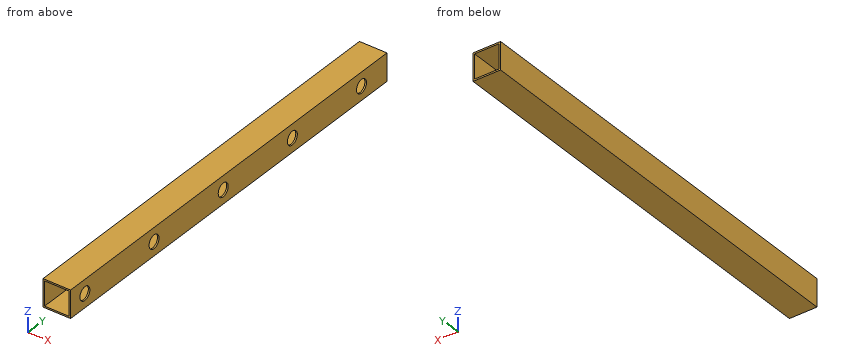
Autodesk Inventor part; units mm, degrees
ref_plane "YZ Plane" through (0, 0, 0) normal (1, 0, 0) x (0, 1, 0)
ref_plane "XZ Plane" through (0, 0, 0) normal (0, 1, 0) x (-1, 0, 0)
ref_plane "XY Plane" through (0, 0, 0) normal (0, 0, 1) x (1, 0, 0)
sketch "Sketch9" plane through (0, 0, 0) normal (0, 1, 0) x (-1, 0, 0)
  line L0 (17.5, 17.5) -> (-17.5, 17.5)
  line L1 (-17.5, 17.5) -> (-17.5, -17.5)
  line L2 (-17.5, -17.5) -> (17.5, -17.5)
  line L3 (17.5, -17.5) -> (17.5, 17.5)
  line L4 (17.5, 17.5) -> (-17.5, -17.5) construction
  line L5 (-17.5, 17.5) -> (17.5, -17.5) construction
  line L6 (-15.5, 15.5) -> (15.5, 15.5)
  line L7 (15.5, 15.5) -> (15.5, -15.5)
  line L8 (15.5, -15.5) -> (-15.5, -15.5)
  line L9 (-15.5, -15.5) -> (-15.5, 15.5)
  point P0 (0, 0)
  dimension "d172" = 35
  dimension "d173" = 35
  dimension "d174" = 2
extrude "Extrusion3" add sketch "Sketch9" against normal blind 540
sketch "Sketch10" plane through (0, 0, 0) normal (1, 0, 0) x (0, 1, 0)
  line L0 (0, 17.5) -> (0, -17.5) construction
  line L1 (0, 17.5) -> (-540, 17.5) construction
  line L2 (-540, -17.5) -> (-540, 17.5) construction
  line L3 (0, -17.5) -> (-540, -17.5) construction
  line L4 (-524, 8.5) -> (-507, 8.5)
  line L5 (-507, 8.5) -> (-507, -8.5)
  line L6 (-507, -8.5) -> (-524, -8.5)
  line L7 (-524, -8.5) -> (-524, 8.5)
  line L8 (-524, 8.5) -> (-507, -8.5) construction
  line L9 (-507, 8.5) -> (-524, -8.5) construction
  circle A0 centre (-515.5, 0) radius 8.5
  line L10 (0, 17.5) -> (0, -17.5)
  point P0 (0, 0)
  point P1 (0, 0)
  point P2 (-540, 0)
  dimension "d177" = 17
  dimension "d178" = 17
  dimension "d191" = 16
extrude "Extrusion4" cut sketch "Sketch10" along normal through all contours A0
pattern_linear "Rectangular Pattern4" count 5 spacing 118 along (0, 1, 0) of "Extrusion4"
properties part number "ANP 1434 FDS WAY tube4" material "Stainless Steel"
Check sheet for the modelled part. Datum: model origin and axes. Units: mm. Give positions to 0.01 mm unless a question says otherwise; leave off trailing zeros. Order: outer loops, then holes, each group sorted by start corner. A loop starts at its lowest first (then second) coordinate and runs counter-clockwise, first axis right, second up. Notation, with made-up numbers: M -16,64.25 L 29,64.25 A24 cw 29,86.25 Z; hole C 81,57.25 d1. An arc over 180 degrees is marked long. Answer in a Markdown table with one row per item. Add a question column.
Q1. Sectioned sample at B-B, the plane z = 0. Record the boundary of the cut face in (x, y).
Q2. Sectioned sample at D-D, the plane y = -279.5. Record the boundary of the cut face in (x, z).
Q3. Gauge pin test, flat end, axial feed: pin 1 Ø10 at (y, z) = (-515.5, 0) entering from +X. Record the tip position at first contact, or that the pin passes through.
Q4. Sectioned sample at A-A, the plane x = 4.5. Record the boundary of the cut face in (y, z).
Q5. Thickness scan on L1, parallel to Y at x = 16.75, z = 0; L2, parallel to X at y = -28, z = 7; L3, parallel to Z at x = 16, y = -397. Record the ranges inside material, lowest first.
Q6. Sectioned sample at C-C, the plane y = -189. Record the boundary of the cut face in (x, z).
Verdict:
| question | item | result |
|---|---|---|
| 1 | outline | M -17.5,-540 L -15.5,-540 L -15.5,0 L -17.5,0 Z; M 15.5,-540 L 17.5,-540 L 17.5,-524 L 15.5,-524 Z; M 15.5,-507 L 17.5,-507 L 17.5,-406 L 15.5,-406 Z; M 15.5,-389 L 17.5,-389 L 17.5,-288 L 15.5,-288 Z; M 15.5,-271 L 17.5,-271 L 17.5,-170 L 15.5,-170 Z; M 15.5,-153 L 17.5,-153 L 17.5,-52 L 15.5,-52 Z; M 15.5,-35 L 17.5,-35 L 17.5,0 L 15.5,0 Z |
| 2 | outline | M -17.5,-17.5 L 17.5,-17.5 L 17.5,-8.5 L 15.5,-8.5 L 15.5,-15.5 L -15.5,-15.5 L -15.5,15.5 L 15.5,15.5 L 15.5,8.5 L 17.5,8.5 L 17.5,17.5 L -17.5,17.5 Z |
| 3 | pin 1 | x = -15.5 |
| 4 | outline | M -540,-17.5 L 0,-17.5 L 0,-15.5 L -540,-15.5 Z; M -540,15.5 L 0,15.5 L 0,17.5 L -540,17.5 Z |
| 5 | L1 | -540 to -524, -507 to -406, -389 to -288, -271 to -170, -153 to -52, -35 to 0 |
| 5 | L2 | -17.5 to -15.5, 15.5 to 17.5 |
| 5 | L3 | -17.5 to -8.49, 8.49 to 17.5 |
| 6 | outline | M -17.5,-17.5 L 17.5,-17.5 L 17.5,17.5 L -17.5,17.5 Z; hole M -15.5,-15.5 L 15.5,-15.5 L 15.5,15.5 L -15.5,15.5 Z |
